For this review, take the finished solid that the model builds, in its own axes (mm). A direction names the side the tool comes from. Coordinates: 2 decimals unless noted, no trailing zeros. Loops run counter-clockwise (first coordinate to the right, second up) from the corner with the lowest first, then second, coordinate; pieces in that order, holes last. Notation, with made-up numbers: (85, 0.25) - (139, 0.25) arc R27 ccw to (139, 18.25) - close; hole circle Ø5 at (40, -36.75). An arc over 180 degrees is marked (long way). Answer as a JSON object with one key per item and string values. Group by question number.
Item 1: We need section A-A (y = 0.95). Give the boundary of the cut face in (x, z), then the cut area to 3 significant figures.
Item 2: We need section C-C (z = 3). Give the boundary of the cut face in (x, y), then the cut area to 3 significant figures.
Item 3: We need section B-B (z = 0). Give the boundary of the cut face in (x, y), then the cut area to 3 significant figures.
Item 4: Tool access review of faces 1 (the flat face through (-0.175, 3.073, -3.362)), 2 (the cylindrical face through (7.301, 2.439, 8.715)): name each direction out of +Z, -Z, +X, -X, +Y, -Y from which nothing blocks a thin tool from reaching the whole face with its end or side.
Item 5: To check wall thickness, follow line 1 (X direction, y = 3.05, z = 0); line 2 (X direction, y = 2.7, z = 5); line 3 (Z direction, x = -1, y = 1.9). State the ranges of each line that lie inside material, in increasing order.
Item 6: We need section D-D (x = 10). Give the boundary of the cut face in (y, z).
Item 7: Clearance check with flat-ended pins moving along their axes: pin 1 (0.9 mm diameter, centred on x = -1.5, y = 1, fed in from +Z); pin 2 (2.5 mm diameter, centred on x = 10, z = 0, fed in from +Y); pin 3 (5 mm diameter, centred on x = -10, z = 0, fed in from +Y). State where each tip first meets the part, or that it passes through.
Item 8: Mouldability with a two-part tool opening along Z and no side actions: class faces 3 (the cylindrical face through (-9.425, 1.852, 1.386)), 4 (the cylindrical face through (-6.715, 1.655, -2.699)), 5 (the cylindrical face through (9.425, 1.852, 1.386)), 6 (the flat face through (0, 1, -11)) as released by +Z, released by -Z, zero draft, split by the parting line, or undercut.
from build123d import *

# Parameters (mm, degrees)
ESQUISSE1_R             = 1.5
BOSS_EXTRU_1_DEPTH      = 10
ENL_V_MAT_EXTRU_1_DEPTH = 20.4229246
CONG_1_R                = 1


with BuildPart() as part:
    # Esquisse1 → Boss.-Extru.1 (new body)
    with BuildSketch(Plane(origin=(0, 0, 0), x_dir=(1, 0, 0), z_dir=(0, 1, 0))):
        Polygon((7, -9), (12.5, -9), (12.5, 11), (0, 11), (0, 3), (7, 3), align=None)
        with Locations(Location((10, 0, 0), (0, 0, 270))):
            Circle(ESQUISSE1_R, mode=Mode.SUBTRACT)
    extrude(amount=BOSS_EXTRU_1_DEPTH)

    # Esquisse2 → Enlèv. mat.-Extru.1 (cut, through all)
    with BuildSketch(Plane(origin=(12.5, 0, 0), x_dir=(0, 0, -1), z_dir=(1, 0, 0))):
        Polygon((-9, 10), (11, 10), (11, 2), (-9, 4.810816694), align=None)
    extrude(amount=-ENL_V_MAT_EXTRU_1_DEPTH, mode=Mode.SUBTRACT)

    # Congé1
    cong_1_edges = [part.edges().sort_by_distance(p)[0] for p in [
        (7, 1.562163339, -3),
        (12.5, 1, -11),
        (12.5, 2.405408347, 9),
        (7, 2.405408347, 9),
    ]]
    fillet(cong_1_edges, radius=CONG_1_R)

    # Symétrie1: part across plane


with BuildPart() as part_1:
    add(part.part)
    add(part.part.mirror(Plane(origin=(0, 10, -11), x_dir=(0, 0, 1), z_dir=(1, 0, 0))))


solid = part_1.part
Check sheet entries:
{
 "1": {"outline": "(-12.5, -10) arc R1 ccw to (-11.5, -11) - (11.5, -11) arc R1 ccw to (12.5, -10) - (12.5, 8) arc R1 ccw to (11.5, 9) - (8, 9) arc R1 ccw to (7, 8) - (7, -2) arc R1 cw to (6, -3) - (-6, -3) arc R1 cw to (-7, -2) - (-7, 8) arc R1 ccw to (-8, 9) - (-11.5, 9) arc R1 ccw to (-12.5, 8) - close; hole circle Ø3 at (-10, 0); hole circle Ø3 at (10, 0)", "area": "317 mm2"},
 "2": {"outline": "(-12.5, 0) - (-7, 0) - (-7, 3.97) - (-12.5, 3.97) - close; (7, 0) - (12.5, 0) - (12.5, 3.97) - (7, 3.97) - close", "area": "43.6 mm2"},
 "3": {"outline": "(-12.5, 0) - (-11.5, 0) - (-11.5, 3.55) - (-12.5, 3.55) - close; (-8.5, 0) - (-7, 0) - (-7, 3.55) - (-8.5, 3.55) - close; (7, 0) - (8.5, 0) - (8.5, 3.55) - (7, 3.55) - close; (11.5, 0) - (12.5, 0) - (12.5, 3.55) - (11.5, 3.55) - close", "area": "17.7 mm2"},
 "4": {"face 1": "-Z, +X, -X, +Y", "face 2": "+Z, +Y, -Y"},
 "5": {"line 1": "x = -12.5 to -11.5, -8.5 to -7, 7 to 8.5, 11.5 to 12.5", "line 2": "x = -12.5 to -7, 7 to 12.5", "line 3": "z = -11 to -3"},
 "6": {"outline": "(0, -11) - (2, -11) - (3.34, -1.5) - (0, -1.5) - close; (0, 1.5) - (3.76, 1.5) - (4.81, 9) - (0, 9) - close"},
 "7": {"pin 1": "stops at z = -3", "pin 2": "passes through", "pin 3": "stops at y = 3.9"},
 "8": {"face 3": "undercut", "face 4": "released by +Z", "face 5": "undercut", "face 6": "released by -Z"}
}
